```python
from build123d import *

# Parameters (mm, degrees)
BOSS_EXTRUDE1_DEPTH = 7.62
SKETCH3_W           = 5.16456173
SKETCH3_H           = 5.178482382
CUT_EXTRUDE2_DEPTH  = 509.122439065
SKETCH4_R           = 2.695407271
SKETCH4_R_2         = 2.747845639
CUT_EXTRUDE3_DEPTH  = 5.08
SKETCH5_R           = 2.274624141
SKETCH5_R_2         = 2.355331531
CUT_EXTRUDE4_DEPTH  = 5.08


with BuildPart() as part:
    # Sketch1 → Boss-Extrude1 (new body)
    with BuildSketch(Plane.XY):
        Polygon((-69.961161881, 0), (438.038838119, 0), (438.038838119, -8.14546996), (-62.055264567, -8.14546996), align=None)
    extrude(amount=BOSS_EXTRUDE1_DEPTH)

    # Sketch3 → Cut-Extrude2 (cut, through all)
    with BuildSketch(Plane(origin=(438.038838119, 0, 0), x_dir=(0, 0, -1), z_dir=(1, 0, 0))):
        with Locations((-3.745160102, -4.144469612)):
            Rectangle(SKETCH3_W, SKETCH3_H)
    extrude(amount=-CUT_EXTRUDE2_DEPTH, mode=Mode.SUBTRACT)

    # Sketch4 → Cut-Extrude3 (cut)
    with BuildSketch(Plane(origin=(0, 0, 0), x_dir=(1, 0, 0), z_dir=(0, 1, 0))):
        with Locations(Location((1.367483079, -3.546323854, 0), (0, 0, 270))):
            Circle(SKETCH4_R)
        with Locations(Location((14.857584748, -3.546323854, 0), (0, 0, 270))):
            Circle(SKETCH4_R_2)
    extrude(amount=-CUT_EXTRUDE3_DEPTH, mode=Mode.SUBTRACT)

    # Sketch5 → Cut-Extrude4 (cut)
    with BuildSketch(Plane.XZ.offset(8.14546996)):
        with Locations((355.642137029, 4.345547061)):
            Circle(SKETCH5_R)
        with Locations((368.018591587, 4.345547061)):
            Circle(SKETCH5_R_2)
    extrude(amount=-CUT_EXTRUDE4_DEPTH, mode=Mode.SUBTRACT)


solid = part.part
```
Here's how the part is built. I have some questions about the finished solid (model axes, mm). Round coordinates to 2 decimals unless told otherwise and drop trailing zeros. Loops run counter-clockwise (first coordinate to the right, second up) from the corner with the lowest first, then second, coordinate; pieces in that order, holes last. Notation, with made-up numbers: (23.5, -36.5) -> (76.5, -36.5) arc R17 cw to (76.5, -24.5) -> close; hole circle Ø1 at (70, 83). An arc over 180 degrees is marked (long way). Answer as CSV lines item,"result". Start each with the question number.
1. If we mould it in two halves opening along X, with no side actions, what happens to faces 1 (the face through (188, -4, 0)), 2 (the face through (-65.95, -4.13, 0.37))? For each: pulls with the +X half, pulls with the -X half, needs draft (parallel to the pull), parting line crosses it, or undercut.
2. I need wall thicknesses on probe 1 along Z at (x, y) = (91, -6); probe 2 along Y at (x, z) = (69, 2.5); probe 3 along X at (y, z) = (-1.25, 5.25). Which ranges of each line are inside material? Lowest first, please. Write a range as from..to.
3. I'm going to push flat-ended pins straight in: P1, Ø3.5, axis at x = 14.86, z = 3.55, coming from the +Y side; P2, Ø1.5, axis at x = 155, z = 4, coming from the +Y side. Where does each tip first touch, or does it pass through?
4. Imagine slicing it at A-A on x = 288. Write out the boundary of the cut face in (y, z).
Solution:
1,face 1,"needs draft"
1,face 2,"pulls with the -X half"
2,probe 1,"0..1.16, 6.33..7.62"
2,probe 2,"-8.15..-6.73, -1.56..0"
2,probe 3,"-68.75..-0.72, 3.46..12.7, 17.01..438.04"
3,P1,"y = -6.73"
3,P2,"y = 0"
4,outline,"(-8.15, 0) -> (0, 0) -> (0, 7.62) -> (-8.15, 7.62) -> close; hole (-6.73, 1.16) -> (-1.56, 1.16) -> (-1.56, 6.33) -> (-6.73, 6.33) -> close"
